Autodesk Inventor part; units mm, degrees
ref_plane "YZ Plane" through (0, 0, 0) normal (1, 0, 0) x (0, 1, 0)
ref_plane "XZ Plane" through (0, 0, 0) normal (0, 1, 0) x (-1, 0, 0)
ref_plane "XY Plane" through (0, 0, 0) normal (0, 0, 1) x (1, 0, 0)
sketch "Boceto1" plane through (0, 0, 0) normal (0, 1, 0) x (-1, 0, 0)
  line L0 (-14.5, -37) -> (14.5, -37)
  line L1 (14.5, -37) -> (14.5, 37)
  line L2 (14.5, 37) -> (-14.5, 37)
  line L3 (-14.5, 37) -> (-14.5, -37)
  line L4 (-14.5, -37) -> (14.5, 37) construction
  line L5 (14.5, -37) -> (-14.5, 37) construction
  line L6 (-2.5, -25) -> (2.5, -25)
  line L7 (2.5, -25) -> (2.5, 25)
  line L8 (2.5, 25) -> (-2.5, 25)
  line L9 (-2.5, 25) -> (-2.5, -25)
  line L10 (-2.5, -25) -> (2.5, 25) construction
  line L11 (2.5, -25) -> (-2.5, 25) construction
  point P0 (0, 0)
  dimension "d2" = 5
  dimension "d3" = 50
  dimension "d4" = 12
  dimension "d5" = 12
extrude "Extrusión1" add sketch "Boceto1" along normal blind 6
sketch "Boceto2" plane through (0, 6, 0) normal (0, 1, 0) x (1, 0, 0)
  circle A0 centre (0, -31) radius 2.35
  line L0 (-14.5, -37) -> (14.5, -37)
  point P0 (0, 0)
  dimension "d8" = 4.7
  dimension "d9" = 6
extrude "Extrusión2" cut sketch "Boceto2" against normal through all
mirror "Simetría1" about plane through (0, 0, 0) normal (0, 0, 1) of "Extrusión2"
properties part number "sotenedor"
Read the model definition and answer for the solid it produces. Units are mm, in the model's axes. A direction names the side the tool comes from. Give positions to 0.01 mm unless a question says otherwise; leave off trailing zeros. Write each loop counter-clockwise with the first axis right and the second up, starting at its lowest first coordinate (ties: lowest second). Pieces come first, ordered by that corner, then holes. Notation, with made-up numbers: (40.5, 13) - (70.5, 13) arc R27 cw to (70.5, 30) - close; hole circle Ø2 at (-39, 33). An arc over 180 degrees is marked (long way). Use CSV: the item, a comma, the result in double quotes. Start each with the question number.
Item 1: The part is cut by section A-A, the plane x = 0. Give the vertices of the cut face in (y, z), and give its area (3 significant figures).
Item 2: The mould has two halves that part along Z. Classify faces 1 (the flat face through (0, 3, 25)), 2 (the flat face through (0, 3, 37)), 3 (the flat face through (-2.5, 3, 0)), 4 (the flat face through (14.5, 3, 1)): pulls with the +Z half, pulls with the -Z half, needs draft (parallel to the pull), parting line crosses it, or undercut.
Item 3: The part is cut by section D-D, the plane z = 22. Give the vertices of the cut face in (x, y).
Item 4: For faces 5 (the flat face through (-3, 0, 1)), 6 (the flat face through (0, 3, -25)), determine the directions among +Z, -Z, +X, -X, +Y, -Y from which every point of the face is accessible in a straight line to the end or side of a thin tool.
Item 5: The part is cut by section B-B, the plane y = 0.95. Give the vertices of the cut face in (x, z), and give its area (3 significant figures).
Item 6: The part is cut by section C-C, the plane z = 31. Give the vertices of the cut face in (x, y), and give its area (3 significant figures).
Item 7: Consider line 1 (Z direction, x = 0, y = 3.9); line 2 (X direction, y = 4.05, z = -31); line 3 (X direction, y = 2.7, z = -14). Determine where each line is inside the solid, lowest interval first.
Taken from the geometry:
1,outline,"(0, -37) - (6, -37) - (6, -33.35) - (0, -33.35) - close; (0, -28.65) - (6, -28.65) - (6, -25) - (0, -25) - close; (0, 25) - (6, 25) - (6, 28.65) - (0, 28.65) - close; (0, 33.35) - (6, 33.35) - (6, 37) - (0, 37) - close"
1,area,"87.6 mm2"
2,face 1,"undercut"
2,face 2,"pulls with the +Z half"
2,face 3,"undercut"
2,face 4,"needs draft"
3,outline,"(-14.5, 0) - (-2.5, 0) - (-2.5, 6) - (-14.5, 6) - close; (2.5, 0) - (14.5, 0) - (14.5, 6) - (2.5, 6) - close"
4,face 5,"+Z, -Z, +X, -X, -Y"
4,face 6,"+Y, -Y"
5,outline,"(-14.5, -37) - (14.5, -37) - (14.5, 37) - (-14.5, 37) - close; hole (-2.5, -25) - (2.5, -25) - (2.5, 25) - (-2.5, 25) - close; hole circle Ø4.7 at (0, -31); hole circle Ø4.7 at (0, 31)"
5,area,"1,860 mm2"
6,outline,"(-14.5, 0) - (-2.35, 0) - (-2.35, 6) - (-14.5, 6) - close; (2.35, 0) - (14.5, 0) - (14.5, 6) - (2.35, 6) - close"
6,area,"146 mm2"
7,line 1,"-37 to -33.35, -28.65 to -25, 25 to 28.65, 33.35 to 37"
7,line 2,"-14.5 to -2.35, 2.35 to 14.5"
7,line 3,"-14.5 to -2.5, 2.5 to 14.5"
